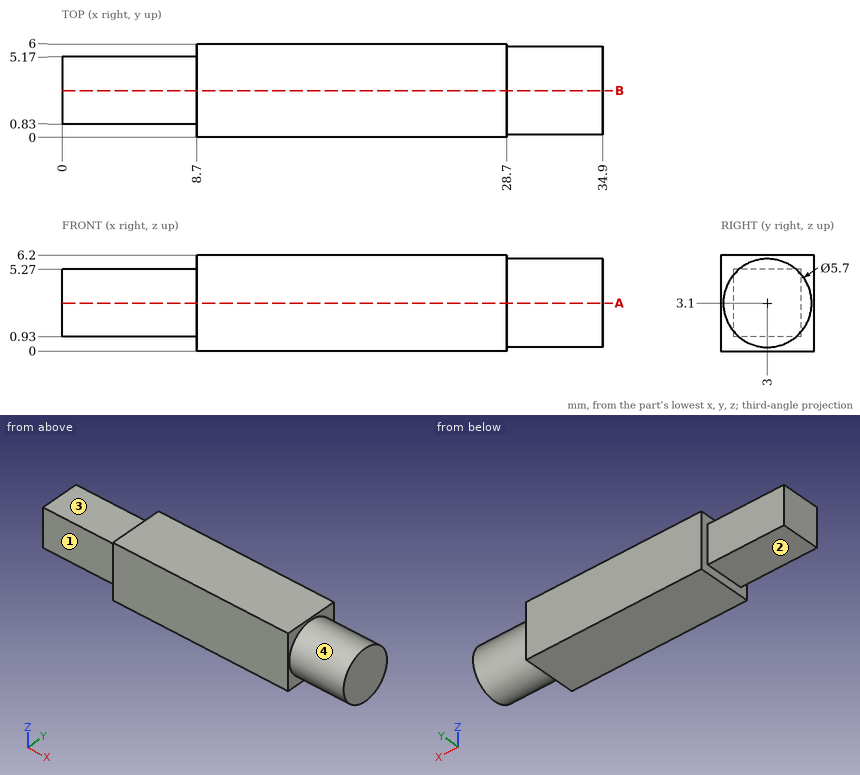
Source: three-view drawing plus pictorial views. Frame: mm from the lowest corner of the part. A direction names the side the tool comes from. Give positions to 0.01 mm unless a question says otherwise; leave off trailing zeros. Order: outer loops, then holes, each group sorted by start corner. A loop starts at its lowest first (then second) coordinate and runs counter-clockwise, first axis right, second up. Notation, with made-up numbers: (59.5, -32.5) - (83.5, -32.5) arc R12 ccw to (83.5, -21.5) - close; hole circle Ø5 at (9, 77.5). An arc over 180 degrees is marked (long way). Put each result on its own line as item: value.
Item 1: Section query A-A, the plane z = 3.1. Return loops of the section in (x, y).
Found:
outline: (0, 0.83) - (8.7, 0.83) - (8.7, 0) - (28.7, 0) - (28.7, 0.15) - (34.9, 0.15) - (34.9, 5.85) - (28.7, 5.85) - (28.7, 6) - (8.7, 6) - (8.7, 5.17) - (0, 5.17) - close
Item 2: Section query B-B, the plane y = 3. Return loops of the section in (x, z).
Found:
outline: (0, 0.93) - (8.7, 0.93) - (8.7, 0) - (28.7, 0) - (28.7, 0.25) - (34.9, 0.25) - (34.9, 5.95) - (28.7, 5.95) - (28.7, 6.2) - (8.7, 6.2) - (8.7, 5.27) - (0, 5.27) - close
Item 3: Ray query, L1, parallel to Y at x = 2.5, z = 4.25; L2, parallel to X at y = 0.8, z = 5.5; L3, parallel to Z at x = 3, y = 1.1. Return the intervals inside material, ascending. Write a range as from..to.
Found:
L1: y = 0.83..5.17
L2: x = 8.7..28.7
L3: z = 0.93..5.27
Item 4: Contact query for flat-ended pins moving along their axis: pin 1 (2 mm diameter, centred on x = 2.5, y = 2.5, fed in from -Z); pin 2 (2 mm diameter, centred on x = 14.5, z = 2, fed in from -Y); pin 3 (3.5 mm diameter, centred on x = 5, y = 2.5, fed in from +Z); pin 4 (1.3 mm diameter, centred on x = 4, z = 3.5, fed in from +Y). Output: stop coordinate, or through.
Found:
pin 1: stops at z = 0.93
pin 2: stops at y = 0
pin 3: stops at z = 5.27
pin 4: stops at y = 5.17
Item 5: Access query for the marked faces 1, 2, 3 and 4. Directions: +Z, -Z, +X, -X, +Y, -Y. A direction counts if a zero-diameter tool reaches every point of the face in a straight line with its end or side. Return the directions, or none.
Found:
face 1: +Z, -Z, -X, -Y
face 2: -Z, -X, +Y, -Y
face 3: +Z, -X, +Y, -Y
face 4: +X
